from build123d import *

# Parameters (mm, degrees)
SKETCH1_W           = 30
SKETCH1_H           = 30
BOSS_EXTRUDE1_DEPTH = 19.05
FILLET1_R           = 4
SKETCH2_R           = 1.5
CUT_EXTRUDE1_DEPTH  = 20.05
SKETCH3_R           = 8.7
BOSS_EXTRUDE2_DEPTH = 32
SKETCH4_R           = 8.7
SKETCH4_R_2         = 6
CUT_EXTRUDE2_DEPTH  = 27


with BuildPart() as part:
    # Sketch1 → Boss-Extrude1 (new body)
    with BuildSketch(Plane.XY):
        Rectangle(SKETCH1_W, SKETCH1_H)
    extrude(amount=BOSS_EXTRUDE1_DEPTH)

    # Fillet1
    fillet1_edges = [part.edges().sort_by_distance(p)[0] for p in [
        (15, -15, 9.525),
        (-15, -15, 9.525),
        (-15, 15, 9.525),
        (15, 15, 9.525),
    ]]
    fillet(fillet1_edges, radius=FILLET1_R)

    # Sketch2 → Cut-Extrude1 (cut, through all)
    with BuildSketch(Plane.XY.offset(19.05)):
        with Locations((-12.2, 12.2)):
            Circle(SKETCH2_R)
        with Locations((12.2, 12.2)):
            Circle(SKETCH2_R)
        with Locations((12.2, -12.2)):
            Circle(SKETCH2_R)
        with Locations((-12.2, -12.2)):
            Circle(SKETCH2_R)
    extrude(amount=-CUT_EXTRUDE1_DEPTH, mode=Mode.SUBTRACT)

    # Sketch3 → Boss-Extrude2 (add)
    with BuildSketch(Plane.XY.offset(19.05)):
        Circle(SKETCH3_R)
    extrude(amount=BOSS_EXTRUDE2_DEPTH)

    # Sketch4 → Cut-Extrude2 (cut)
    with BuildSketch(Plane.XY.offset(19.05)):
        Circle(SKETCH4_R)
        Circle(SKETCH4_R_2, mode=Mode.SUBTRACT)
    extrude(amount=CUT_EXTRUDE2_DEPTH, mode=Mode.SUBTRACT)


solid = part.part
Read the model definition and answer for the solid it produces. Units are mm, in the model's axes. A direction names the side the tool comes from. Give positions to 0.01 mm unless a question says otherwise; leave off trailing zeros. Write each loop counter-clockwise with the first axis right and the second up, starting at its lowest first coordinate (ties: lowest second). Pieces come first, ordered by that corner, then holes. Notation, with made-up numbers: (9.5, 88) - (34.5, 88) arc R15 cw to (34.5, 104) - close; hole circle Ø5 at (24.5, 51). An arc over 180 degrees is marked (long way). Answer in a Markdown table with one row per item. Add a question column.
Item 1: Section A-A, the plane z = 12.5 is taken. Write down the section's boundary in (x, y), and give its area (3 significant figures).
Item 2: Find the intervals of material crossed by L1, parallel to Y at x = 12.2, z = 11; L2, parallel to Z at x = -6.75, y = -3.75; L3, parallel to Y at x = -12.75, z = 16.5, in increasing order.
Item 3: Section B-B, the plane x = 12.75 is taken. Write down the section's boundary in (y, z), and give its area (3 significant figures).
Item 4: Section D-D, the plane y = 0 is taken. Write down the section's boundary in (x, z), and give its area (4 significant figures).
Item 5: Flat-ended cylindrical pins translate along their axes: P1, Ø12, axis at x = 9, z = 27, coming from the -Y side; P2, Ø2, axis at x = -5, z = 21.5, coming from the +Y side; P3, Ø8, axis at y = -9.5, z = 25.5, coming from the +X side. Find the tip coordinate at first contact, or state that the pin passes through.
Item 6: Determine the mould class of faces 1 (the face through (-10.814, -12.775, 9.658)), 2 (the face through (-13.859, 13.797, 9.658)), 3 (the face through (0, 15, 9)) for opening direction X: pulls with the +X half, pulls with the -X half, needs draft (parallel to the pull), parting line crosses it, or undercut.
Item 7: Section C-C, the plane y = 12.2 is taken. Write down the section's boundary in (x, z), and give its area (3 significant figures).
Item 8: A tool of negligible diameter and unlimited length cuts with its end or side. For faces 4 (the face through (0, -15, 9)), 5 (the face through (-1.886, -8.493, 48.515)), 6 (the face through (-6, 0, 32)), from which of +Z, -Z, +X, -X, +Y, -Y can it reach the whole face along a straight path? Write none if from no direction.
Recorded:
| question | item | result |
|---|---|---|
| 1 | outline | (-15, -11) arc R4 ccw to (-11, -15) - (11, -15) arc R4 ccw to (15, -11) - (15, 11) arc R4 ccw to (11, 15) - (-11, 15) arc R4 ccw to (-15, 11) - close; hole circle Ø3 at (-12.2, -12.2); hole circle Ø3 at (-12.2, 12.2); hole circle Ø3 at (12.2, -12.2); hole circle Ø3 at (12.2, 12.2) |
| 1 | area | 858 mm2 |
| 2 | L1 | y = -14.82 to -13.7, -10.7 to 10.7, 13.7 to 14.82 |
| 2 | L2 | z = 0 to 19.05, 46.05 to 51.05 |
| 2 | L3 | y = -14.6 to -13.6, -10.8 to 10.8, 13.6 to 14.6 |
| 3 | outline | (-14.6, 0) - (-13.6, 0) - (-13.6, 19.05) - (-14.6, 19.05) - close; (-10.8, 0) - (10.8, 0) - (10.8, 19.05) - (-10.8, 19.05) - close; (13.6, 0) - (14.6, 0) - (14.6, 19.05) - (13.6, 19.05) - close |
| 3 | area | 450 mm2 |
| 4 | outline | (-15, 0) - (15, 0) - (15, 19.05) - (6, 19.05) - (6, 46.05) - (8.7, 46.05) - (8.7, 51.05) - (-8.7, 51.05) - (-8.7, 46.05) - (-6, 46.05) - (-6, 19.05) - (-15, 19.05) - close |
| 4 | area | 982.5 mm2 |
| 5 | P1 | stops at y = -5.2 |
| 5 | P2 | stops at y = 4.47 |
| 5 | P3 | stops at x = 2.4 |
| 6 | face 1 | undercut |
| 6 | face 2 | pulls with the -X half |
| 6 | face 3 | needs draft |
| 7 | outline | (-14.82, 0) - (-13.7, 0) - (-13.7, 19.05) - (-14.82, 19.05) - close; (-10.7, 0) - (10.7, 0) - (10.7, 19.05) - (-10.7, 19.05) - close; (13.7, 0) - (14.82, 0) - (14.82, 19.05) - (13.7, 19.05) - close |
| 7 | area | 450 mm2 |
| 8 | face 4 | +Z, -Z, +X, -X, -Y |
| 8 | face 5 | +Z |
| 8 | face 6 | none |
